Model file for the job. Use its own axes, mm. A direction names the side the tool comes from. Coordinates: 2 decimals unless noted, no trailing zeros. Loops run counter-clockwise (first coordinate to the right, second up) from the corner with the lowest first, then second, coordinate; pieces in that order, holes last. Notation, with made-up numbers: (13.25, 67) -> (41.25, 67) arc R22 ccw to (41.25, 93) -> close; hole circle Ø9 at (-16, 29.25). An arc over 180 degrees is marked (long way). Use one line per item in the form item = value.
```python
from build123d import *

# Parameters (mm, degrees)
BOX033_W               = 80
BOX033_H               = 4
BOX033_DEPTH           = 80
BOX033_PLACEMENT_ANGLE = 45
FILLET130_R            = 20
BOX035_W               = 80
BOX035_H               = 4
BOX035_DEPTH           = 80
BOX035_PLACEMENT_ANGLE = 45
FILLET131_R            = 20
BOX036_W               = 120
BOX036_H               = 4
BOX036_DEPTH           = 120
BOX036_PLACEMENT_ANGLE = 45
FILLET133_R            = 60
CYLINDER090_R          = 1.6
CYLINDER090_DEPTH      = 25
CYLINDER091_R          = 1.6
CYLINDER091_DEPTH      = 25
CYLINDER092_R          = 1.6
CYLINDER092_DEPTH      = 25
CYLINDER089_R          = 1.6
CYLINDER089_DEPTH      = 25
BOX034_W               = 100
BOX034_H               = 4
BOX034_DEPTH           = 100
BOX034_PLACEMENT_ANGLE = 45
FILLET132_R            = 60
BOX032_W               = 148
BOX032_H               = 4
BOX032_DEPTH           = 200
FILLET134_R            = 30
FILLET135_R            = 10
CHAMFER035_SIZE        = 2


with BuildPart() as fillet131:
    # Box033 → Box033 (new body)
    with BuildSketch(Plane.XY):
        with Locations((40, 2)):
            Rectangle(BOX033_W, BOX033_H)
    extrude(amount=BOX033_DEPTH)


with BuildPart() as fillet131_1:
    # Box033 placement: moved
    add(fillet131.part.moved(Location((-6.57, 0, 202))).rotate(Axis((-6.57, 0, 202), (0, 1, 0)), BOX033_PLACEMENT_ANGLE))

    # Fillet130
    fillet130_edges = [fillet131_1.edges().sort_by_distance(p)[0] for p in [
        (49.998542, 2, 145.431458),
    ]]
    fillet(fillet130_edges, radius=FILLET130_R)


with BuildPart() as fillet132:
    # Box035 → Box035 (new body)
    with BuildSketch(Plane.XY):
        with Locations((40, 2)):
            Rectangle(BOX035_W, BOX035_H)
    extrude(amount=BOX035_DEPTH)


with BuildPart() as fillet132_1:
    # Box035 placement: moved
    add(fillet132.part.moved(Location((-6.57, 0, -2))).rotate(Axis((-6.57, 0, -2), (0, 1, 0)), BOX035_PLACEMENT_ANGLE))

    # Fillet131
    fillet131_edges = [fillet132_1.edges().sort_by_distance(p)[0] for p in [
        (49.998542, 2, 54.568542),
    ]]
    fillet(fillet131_edges, radius=FILLET131_R)


with BuildPart() as fillet134:
    # Box036 → Box036 (new body)
    with BuildSketch(Plane.XY):
        with Locations((60, 2)):
            Rectangle(BOX036_W, BOX036_H)
    extrude(amount=BOX036_DEPTH)


with BuildPart() as fillet134_1:
    # Box036 placement: moved
    add(fillet134.part.moved(Location((48.67, 0, 100))).rotate(Axis((48.67, 0, 100), (0, 1, 0)), BOX036_PLACEMENT_ANGLE))

    # Fillet133
    fillet133_edges = [fillet134_1.edges().sort_by_distance(p)[0] for p in [
        (48.67, 2, 100),
    ]]
    fillet(fillet133_edges, radius=FILLET133_R)


with BuildPart() as obj1:
    # Cylinder090 → Cylinder090 (new body)
    with BuildSketch(Plane(origin=(125, -20, 15), x_dir=(1, 0, 0), z_dir=(0, 1, 0))):
        Circle(CYLINDER090_R)
    extrude(amount=CYLINDER090_DEPTH)


with BuildPart() as obj2:
    # Cylinder091 → Cylinder091 (new body)
    with BuildSketch(Plane(origin=(-13, -20, 193), x_dir=(1, 0, 0), z_dir=(0, 1, 0))):
        Circle(CYLINDER091_R)
    extrude(amount=CYLINDER091_DEPTH)


with BuildPart() as obj3:
    # Cylinder092 → Cylinder092 (new body)
    with BuildSketch(Plane(origin=(125, -20, 193), x_dir=(1, 0, 0), z_dir=(0, 1, 0))):
        Circle(CYLINDER092_R)
    extrude(amount=CYLINDER092_DEPTH)


with BuildPart() as obj4:
    # Cylinder089 → Cylinder089 (new body)
    with BuildSketch(Plane(origin=(-13, -20, 15), x_dir=(1, 0, 0), z_dir=(0, 1, 0))):
        Circle(CYLINDER089_R)
    extrude(amount=CYLINDER089_DEPTH)

    # Fusion055: union obj1, obj2, obj3
    add(obj1.part)
    add(obj2.part)
    add(obj3.part)


with BuildPart() as fusion056:
    # Box034 → Box034 (new body)
    with BuildSketch(Plane.XY):
        with Locations((50, 2)):
            Rectangle(BOX034_W, BOX034_H)
    extrude(amount=BOX034_DEPTH)


with BuildPart() as fusion056_1:
    # Box034 placement: moved
    add(fusion056.part.moved(Location((-90, 0, 100))).rotate(Axis((-90, 0, 100), (0, 1, 0)), BOX034_PLACEMENT_ANGLE))

    # Fillet132
    fillet132_edges = [fusion056_1.edges().sort_by_distance(p)[0] for p in [
        (51.421356, 2, 100),
    ]]
    fillet(fillet132_edges, radius=FILLET132_R)

    # Fusion056: union Fillet131, Fillet132, Fillet134, obj4
    add(fillet131_1.part)
    add(fillet132_1.part)
    add(fillet134_1.part)
    add(obj4.part)


with BuildPart() as support2:
    # Box032 → Box032 (new body)
    with BuildSketch(Plane(origin=(-18, 0, 0), x_dir=(1, 0, 0), z_dir=(0, 0, 1))):
        with Locations((74, 2)):
            Rectangle(BOX032_W, BOX032_H)
    extrude(amount=BOX032_DEPTH)

    # Cut017: cut Fusion056
    add(fusion056_1.part, mode=Mode.SUBTRACT)

    # Fillet134
    fillet134_edges = [support2.edges().sort_by_distance(p)[0] for p in [
        (-18, 2, 30.578644),
        (-18, 2, 169.421356),
    ]]
    fillet(fillet134_edges, radius=FILLET134_R)

    # Fillet135
    fillet135_edges = [support2.edges().sort_by_distance(p)[0] for p in [
        (130, 2, 181.33),
        (130, 2, 18.67),
    ]]
    fillet(fillet135_edges, radius=FILLET135_R)

    # Chamfer035
    chamfer035_edges = [support2.edges().sort_by_distance(p)[0] for p in [
        (-14.6, 0, 15),
        (-14.6, 0, 193),
        (123.4, 0, 15),
        (123.4, 0, 193),
    ]]
    chamfer(chamfer035_edges, length=CHAMFER035_SIZE)


solid = support2.part
```
Q1. Band-saw the part on D-D, the plane z = 145. Write the cut outline in (x, y), and give its area (3 significant figures).
Result:
outline = (6.42, 0) -> (93.67, 0) -> (93.67, 4) -> (6.42, 4) -> close
area = 349 mm2
Q2. Wall check: line 1 along Z through (x, y) = (125, 2.7); line 2 along X through (y, z) = (3.3, 193); line 3 along Z through (x, y) = (-13, 3.25). Give the ranges that are in metal, low to high.
Result:
line_1 = 0 to 13.4, 16.6 to 23.67, 176.33 to 191.4, 194.6 to 200
line_2 = -18 to -14.6, -11.4 to 2.43, 97.57 to 123.4, 126.6 to 130
line_3 = 0 to 13.4, 16.6 to 34.74, 165.26 to 191.4, 194.6 to 200
Q3. Mould opens along Z. For faces 1 (the face through (-15.78, 2.03, 29.48)), 2 (the face through (50.218, 2.028, 153.717)), 3 (the face through (117, 2, 0)), 4 (the face through (129.218, 2.028, 18.405)) say: released by +Z, released by -Z, zero draft, split by the parting line, or undercut.
Result:
face_1 = undercut
face_2 = released by +Z
face_3 = released by -Z
face_4 = undercut
Q4. Pin check, flat tips, straight feed: pin 1 Ø1.9 at (x, z) = (-13, 15) entering from +Y; pin 2 Ø1.5 at (y, z) = (1.5, 168) entering from -X; pin 3 Ø2 at (y, z) = (2.5, 81.5) entering from -X; pin 4 Ø2 at (y, z) = (0.5, 95) entering from +X. Stop position of each tip, or through.
Result:
pin_1 = through
pin_2 = -14.99
pin_3 = 23.31
pin_4 = 73.82
Q5. Band-saw the part on B-B, the plane y = 1. Write the cut outline in (x, z).
Result:
outline = (-18, 0) -> (-4.57, 0) -> (35.86, 40.43) arc R20 cw to (64.14, 40.43) -> (104.57, 0) -> (130, 0) -> (130, 14.53) arc R10 ccw to (127.07, 21.6) -> (91.1, 57.57) arc R60 cw to (91.1, 142.43) -> (127.07, 178.4) arc R10 ccw to (130, 185.47) -> (130, 200) -> (104.57, 200) -> (64.14, 159.57) arc R20 cw to (35.86, 159.57) -> (-4.57, 200) -> (-18, 200) -> (-18, 181.85) arc R30 ccw to (-9.21, 160.63) -> (8.99, 142.43) arc R60 cw to (8.99, 57.57) -> (-9.21, 39.37) arc R30 ccw to (-18, 18.15) -> close; hole circle Ø5.2 at (-13, 15); hole circle Ø5.2 at (-13, 193); hole circle Ø5.2 at (125, 15); hole circle Ø5.2 at (125, 193)
Q6. Which spindle directions (+Z, -Z, +X, -X, +Y, -Y) get a long thin tool onto all of the face, cutting with end or side? Do faces 5 (the face through (15.36, 2.03, 180.07)), 6 (the face through (15.36, 1.97, 19.93)), 7 (the face through (-0.24, 2.03, 151.66)), 8 (the face through (108.83, 2.03, 39.84)). Say none if no direction does.
Result:
face_5 = +Z, +Y, -Y
face_6 = -Z, +Y, -Y
face_7 = -X, +Y, -Y
face_8 = +X, +Y, -Y
Q7. Band-saw the part on C-C, the plane x = 78. Write the cut outline in (y, z), and give its area (3 significant figures).
Result:
outline = (0, 26.57) -> (4, 26.57) -> (4, 77.26) -> (0, 77.26) -> close; (0, 122.74) -> (4, 122.74) -> (4, 173.43) -> (0, 173.43) -> close
area = 406 mm2
Q8. Band-saw the part on A-A, the plane x = 117. Write the cut outline in (y, z), and give its area (3 significant figures).
Result:
outline = (0, 0) -> (4, 0) -> (4, 31.67) -> (0, 31.67) -> close; (0, 168.33) -> (4, 168.33) -> (4, 200) -> (0, 200) -> close
area = 253 mm2
